```python
from build123d import *

# Parameters (mm, degrees)
SKETCH_1_R          = 6
EXTRUDE_1_DEPTH     = 54
FILLET_1_R          = 6
SKETCH_2_W          = 76
SKETCH_2_H          = 26
CUT_EXTRUDE_1_DEPTH = 83
CUT_EXTRUDE_2_REACH = 178


with BuildPart() as part:
    # 스케치1 → 보스-돌출1 (new body)
    with BuildSketch(Plane(origin=(0, 0, 0), x_dir=(1, 0, 0), z_dir=(0, 1, 0))):
        Polygon((0, 32), (68, 32), (68, 82), (176, 82), (176, 50), (100, 50), (100, 0), (0, 0), align=None)
        with Locations(Location((116, 66, 0), (0, 0, 270))):  # turned: the seam where the file's is
            Circle(SKETCH_1_R, mode=Mode.SUBTRACT)
        with Locations(Location((160, 66, 0), (0, 0, 270))):  # turned: the seam where the file's is
            Circle(SKETCH_1_R, mode=Mode.SUBTRACT)
    extrude(amount=EXTRUDE_1_DEPTH)

    # 필렛1
    fillet_1_edges = [part.edges().sort_by_distance(p)[0] for p in [
        (68, 27, -32),
        (100, 27, -50),
    ]]
    fillet(fillet_1_edges, radius=FILLET_1_R)

    # 스케치2 → 컷-돌출1 (cut, through all)
    with BuildSketch(Plane.XY):
        with BuildLine():
            Line((87, 35), (87, 15))
            Line((87, 15), (176, 15))
            Line((176, 15), (176, 0))
            Line((176, 0), (13, 0))
            Line((13, 0), (13, 35))
            ThreePointArc((13, 35), (14.757359313, 39.242640687), (19, 41))
            Line((19, 41), (81, 41))
            ThreePointArc((81, 41), (85.242640687, 39.242640687), (87, 35))
        make_face()
        with Locations((138, 41)):
            Rectangle(SKETCH_2_W, SKETCH_2_H)
    extrude(amount=-CUT_EXTRUDE_1_DEPTH, mode=Mode.SUBTRACT)

    # 스케치3 → 컷-돌출2 (cut, up to next)
    with BuildSketch(Plane(origin=(0, 0, 0), x_dir=(0, 0, -1), z_dir=(1, 0, 0)), mode=Mode.PRIVATE) as cut_extrude_2_sk1:
        with BuildLine():
            Line((23, 15), (23, 0))
            Line((23, 0), (9, 0))
            Line((9, 0), (9, 15))
            ThreePointArc((9, 15), (16, 22), (23, 15))
        make_face()
    cut_extrude_2_tool1 = extrude(cut_extrude_2_sk1.sketch, amount=CUT_EXTRUDE_2_REACH, mode=Mode.PRIVATE) & part.part
    add(cut_extrude_2_tool1.solids().sort_by_distance((0, 10.308437, -16))[0], mode=Mode.SUBTRACT)


solid = part.part
```
Source: CAD feature listing. Evaluate the final solid. Frame: model axes, mm. A direction names the side the tool comes from. Give positions to 0.01 mm unless a question says otherwise; leave off trailing zeros. Loops run counter-clockwise (first coordinate to the right, second up) from the corner with the lowest first, then second, coordinate; pieces in that order, holes last. Notation, with made-up numbers: (37, 0) -> (88, 0) arc R17 cw to (88, 8) -> close; hole circle Ø9 at (-9.75, 80). An arc over 180 degrees is marked (long way). Put each result on its own line as item: value. Start each with the question number.
1) Draft query along Z for faces 1 (the face through (17, 45, -32)), 2 (the face through (6, 22, -16)), 3 (the face through (68, 47, -60)). Return one class per face: released by +Z, released by -Z, zero draft, split by the parting line, or undercut.
2) Reachability of faces 4 (the face through (141, 21, -50)), 5 (the face through (6, 7, -9)), 6 (the face through (56, 41, -22)), 7 (the face through (100, 39, -42)), 8 (the face through (137, 28, -63)) from +Z, -Z, +X, -X, +Y, -Y: full face, straight path, thin tool, end or side. Return the list, or none.
3) Material intervals for probe 1 along X at (y, z) = (21.5, -66); probe 2 along Z at (x, y) = (116, 22.25); probe 3 along X at (y, z) = (29, -15), sorted ascending.
4) Cut plane C-C (x = 116). Return loops of the section in (y, z), then the cut area to 3 significant figures.
5) Contact query for flat-ended pins moving along their axis: P1, Ø3, axis at y = 42.5, z = -70, coming from the +X side; P2, Ø6.5, axis at x = 8.5, y = 7.5, coming from the -Z side; P3, Ø11.5, axis at x = 127.5, z = -61.5, coming from the +Y side; P4, Ø3, axis at x = 67.5, y = 42, coming from the +Z side. Output: stop coordinate, or through.
6) Cut plane D-D (y = 38). Return loops of the section in (x, z), then the cut area to 3 significant figures.
7) Cut plane B-B (z = -66). Return loops of the section in (x, y).
8) Cut plane A-A (y = 25.5). Return loops of the section in (x, z).
Results are:
1. face 1: released by -Z
1. face 2: undercut
1. face 3: zero draft
2. face 4: +Z, +X, +Y, -Y
2. face 5: +X, -X, -Y
2. face 6: +Z, -Z, -Y
2. face 7: +Z, +X, +Y
2. face 8: +Z, -Z, +X, +Y
3. probe 1: x = 87 to 110, 122 to 154, 166 to 176
3. probe 2: z = -82 to -72, -60 to -50
3. probe 3: x = 0 to 13, 87 to 100
4. outline: (15, -82) -> (28, -82) -> (28, -72) -> (15, -72) -> close; (15, -60) -> (28, -60) -> (28, -50) -> (15, -50) -> close
4. area: 260 mm2
5. P1: stops at x = 100
5. P2: stops at z = -32
5. P3: stops at y = 28
5. P4: stops at z = 0
6. outline: (0, -32) -> (13.8, -32) -> (13.8, 0) -> (0, 0) -> close; (86.2, -82) -> (100, -82) -> (100, 0) -> (86.2, 0) -> close
6. area: 1,570 mm2
7. outline: (68, 41) -> (81, 41) arc R6 cw to (87, 35) -> (87, 15) -> (110, 15) -> (110, 28) -> (100, 28) -> (100, 54) -> (68, 54) -> close; (122, 15) -> (154, 15) -> (154, 28) -> (122, 28) -> close; (166, 15) -> (176, 15) -> (176, 28) -> (166, 28) -> close
8. outline: (0, -32) -> (13, -32) -> (13, 0) -> (0, 0) -> close; (87, -82) -> (176, -82) -> (176, -50) -> (106, -50) arc R6 cw to (100, -44) -> (100, 0) -> (87, 0) -> close; hole circle Ø12 at (116, -66); hole circle Ø12 at (160, -66)
